Build history of the part. All positions in model axes, mm. Face numbers are marked on the shaded views. A direction names the side the tool comes from. Give positions to 0.01 mm unless a question says otherwise; leave off trailing zeros. Order: outer loops, then holes, each group sorted by start corner. A loop starts at its lowest first (then second) coordinate and runs counter-clockwise, first axis right, second up. Notation, with made-up numbers: M 70,-19.75 L 126,-19.75 A14 cw 126,-11.75 Z; hole C 62,-3 d11. An arc over 180 degrees is marked long. Answer as CSV lines item,"result".
from build123d import *

# Parameters (mm, degrees)
SKETCH_1_W             = 40
SKETCH_1_H             = 34
SKETCH_1_R             = 5.5
EXTRUDE_1_DEPTH        = 10
CUT_EXTRUDE_2_DEPTH    = 29.08914381
FILLET_1_R             = 1
HOLE_WIZARD_M3_1_D     = 2.5
SKETCH_13_W            = 40
SKETCH_13_H            = 9.5
EXTRUDE_2_DEPTH        = 10
HOLE_WIZARD_M4_1_D     = 3.3
HOLE_WIZARD_M4_1_DEPTH = 14.5
HOLE_WIZARD_M4_3_D     = 3.3


with BuildPart() as part:
    # 草图1 → 凸台-拉伸1 (new body)
    with BuildSketch(Plane(origin=(0, 0, 0), x_dir=(1, 0, 0), z_dir=(0, 1, 0))):
        Rectangle(SKETCH_1_W, SKETCH_1_H)
        with Locations(Location((0, 0, 0), (0, 0, 270))):
            Circle(SKETCH_1_R, mode=Mode.SUBTRACT)
    extrude(amount=EXTRUDE_1_DEPTH)

    # 草图3 → 切除-拉伸2 (cut, through all)
    with BuildSketch(Plane.XZ):
        with BuildLine():
            Line((-36.5, -12), (-4.5, -12))
            ThreePointArc((-4.5, -12), (-3.792893219, -11.707106781), (-3.5, -11))
            Line((-3.5, -11), (-3.5, 11))
            ThreePointArc((-3.5, 11), (-3.792893219, 11.707106781), (-4.5, 12))
            Line((-4.5, 12), (-36.5, 12))
            Line((-36.5, 12), (-36.5, -12))
        make_face()
        with BuildLine():
            Line((12, -12), (29, -12))
            Line((29, -12), (29, 12))
            Line((29, 12), (12, 12))
            ThreePointArc((12, 12), (11.292893219, 11.707106781), (11, 11))
            Line((11, 11), (11, -11))
            ThreePointArc((11, -11), (11.292893219, -11.707106781), (12, -12))
        make_face()
    extrude(amount=-CUT_EXTRUDE_2_DEPTH, mode=Mode.SUBTRACT)

    # 圆角1
    fillet_1_edges = [part.edges().sort_by_distance(p)[0] for p in [
        (-20, 5, -12),
        (-20, 5, 12),
        (20, 5, 12),
        (20, 5, -12),
    ]]
    fillet(fillet_1_edges, radius=FILLET_1_R)

    # M3 螺纹孔1 (through all)
    with Locations(Plane.ZY.offset(3.5)):
        with Locations((-8.5, 5), (8.5, 5)):
            Hole(HOLE_WIZARD_M3_1_D / 2)

    # 草图13 → 凸台-拉伸2 (add)
    with BuildSketch(Plane(origin=(0, 0, 0), x_dir=(-1, 0, 0), z_dir=(0, -1, 0))):
        with Locations((0, -21.75)):
            Rectangle(SKETCH_13_W, SKETCH_13_H)
    extrude(amount=-EXTRUDE_2_DEPTH)

    # M4 螺纹孔1
    with Locations(Plane.XY.offset(26.5)):
        with Locations((-15, 5), (15, 5)):
            Hole(HOLE_WIZARD_M4_1_D / 2, depth=HOLE_WIZARD_M4_1_DEPTH)

    # M4 螺纹孔3 (through all)
    with Locations(Plane(origin=(15, 5, -17), x_dir=(-1, 0, 0), z_dir=(0, 0, -1))):
        with Locations((0, 0), (30, 0)):
            Hole(HOLE_WIZARD_M4_3_D / 2)


solid = part.part
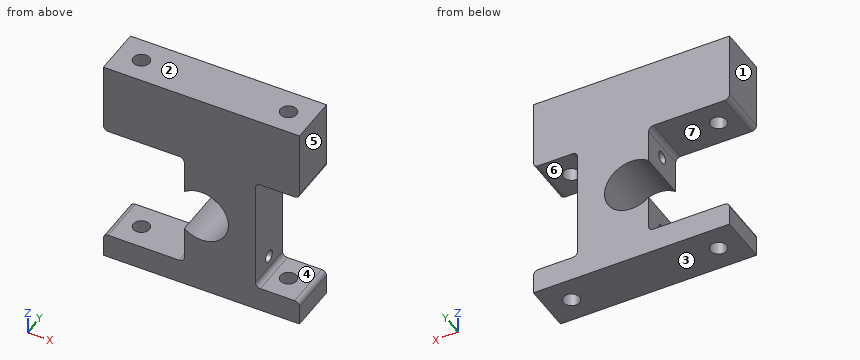
Item 1: Band-saw the part on A-A (x = 0). Give the cut face in (y, z).
Geometry says:
outline,"M 0,-17 L 10,-17 L 10,-5.5 L 0,-5.5 Z; M 0,5.5 L 10,5.5 L 10,26.5 L 0,26.5 Z; hole C 5,-8.5 d2.5; hole C 5,8.5 d2.5"
Item 2: Probe line 1 along Y through (x, z) = (15, 21.25); line 2 along Z through (x, y) = (-4.5, 7); line 3 along Z through (x, y) = (1, 5.5). List the from-to ranges inside material, lowest first. Write a range as from..to.
Geometry says:
line 1,"y = 0..3.35, 6.65..10"
line 2,"z = -17..-12, 12..26.5"
line 3,"z = -17..-9.65, -7.35..-5.41, 5.41..7.35, 9.65..26.5"
Item 3: Band-saw the part on B-B (z = 8.5). Give the cut face in (x, y), and give its area (3 significant figures).
Geometry says:
outline,"M -3.5,0 L 11,0 L 11,3.75 L -3.5,3.75 Z; M -3.5,6.25 L 11,6.25 L 11,10 L -3.5,10 Z"
area,"109 mm2"
Item 4: Band-saw the part on D-D (x = -8.5). Give the cut face in (y, z).
Geometry says:
outline,"M 0,-17 L 10,-17 L 10,-12 L 0,-12 Z; M 0,12 L 10,12 L 10,26.5 L 0,26.5 Z"
Item 5: Drop flat-ended pins along their axis: pin 1 (4 mm diameter, centred on y = 2, z = -1, fed in from -X); pin 2 (2.5 mm diameter, centred on x = 15, y = 5, fed in from +Z); pin 3 (3.5 mm diameter, centred on y = 6, z = 8, fed in from -X); pin 4 (3 mm diameter, centred on y = 3, z = -1, fed in from +X). Give the stop position or say it passes through.
Geometry says:
pin 1,"stops at x = 4.61"
pin 2,"passes through"
pin 3,"stops at x = -3.5"
pin 4,"stops at x = 11"
Item 6: 3-axis set-ups, long thin cutter, end or side, ignore diameter. For the marked faces 5, 6 and 7: which of +Z, -Z, +X, -X, +Y, -Y reach the whole face in a straight line?
Geometry says:
face 5,"+Z, -Z, +X, +Y, -Y"
face 6,"+X, +Y, -Y"
face 7,"-X, +Y, -Y"
Item 7: Pull direction Z, two halves, no side cores. Call the marked faces 1, 2, 3 and 4: released by +Z, released by -Z, zero draft, split by the parting line, or undercut.
Geometry says:
face 1,"zero draft"
face 2,"released by +Z"
face 3,"released by -Z"
face 4,"undercut"
Item 8: Band-saw the part on C-C (x = 15). Give the cut face in (y, z).
Geometry says:
outline,"M 0,-17 L 3.35,-17 L 3.35,-12 L 0,-12 Z; M 0,12 L 3.35,12 L 3.35,26.5 L 0,26.5 Z; M 6.65,-17 L 10,-17 L 10,-12 L 6.65,-12 Z; M 6.65,12 L 10,12 L 10,26.5 L 6.65,26.5 Z"
